Here's how the part is built. I have some questions about the finished solid (model axes, mm). Face numbers are marked on the shaded views. A direction names the side the tool comes from. Coordinates: 2 decimals unless noted, no trailing zeros. Write each loop counter-clockwise with the first axis right and the second up, starting at its lowest first coordinate (ties: lowest second). Pieces come first, ordered by that corner, then holes. Notation, with made-up numbers: M 79.5,-34.75 L 103.5,-34.75 A21 cw 103.5,-23.75 Z; hole C 76,1 d11. An arc over 180 degrees is marked long. Write each question's results on one line, items separated by ' | '. Start each with the question number.
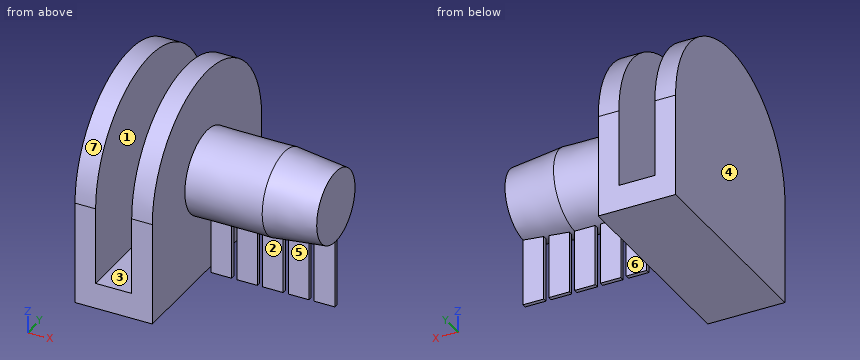
from build123d import *

# Parameters (mm, degrees)
BOX002004_W           = 4
BOX002004_H           = 0.8
BOX002004_DEPTH       = 13
BOX002003_W           = 4
BOX002003_H           = 0.8
BOX002003_DEPTH       = 13
BOX002002_W           = 4
BOX002002_H           = 0.8
BOX002002_DEPTH       = 13
BOX002001_W           = 4
BOX002001_H           = 0.8
BOX002001_DEPTH       = 13
BOX002_W              = 4
BOX002_H              = 0.8
BOX002_DEPTH          = 13
BOX001_W              = 36
BOX001_H              = 46
BOX001_DEPTH          = 7
CYLINDER001_R         = 20
CYLINDER001_DEPTH     = 15
BOX_W                 = 20
BOX_H                 = 40
BOX_DEPTH             = 15
FUSION002_PITCH_ANGLE = 90


with BuildPart() as support005:
    # Box002004 → Box002004 (new body)
    with BuildSketch(Plane(origin=(36, -0.4, -20), x_dir=(1, 0, 0), z_dir=(0, 0, 1))):
        with Locations((2, 0.4)):
            Rectangle(BOX002004_W, BOX002004_H)
    extrude(amount=BOX002004_DEPTH)


with BuildPart() as support004:
    # Box002003 → Box002003 (new body)
    with BuildSketch(Plane(origin=(31, -0.4, -20), x_dir=(1, 0, 0), z_dir=(0, 0, 1))):
        with Locations((2, 0.4)):
            Rectangle(BOX002003_W, BOX002003_H)
    extrude(amount=BOX002003_DEPTH)


with BuildPart() as support003:
    # Box002002 → Box002002 (new body)
    with BuildSketch(Plane(origin=(26, -0.4, -20), x_dir=(1, 0, 0), z_dir=(0, 0, 1))):
        with Locations((2, 0.4)):
            Rectangle(BOX002002_W, BOX002002_H)
    extrude(amount=BOX002002_DEPTH)


with BuildPart() as support002:
    # Box002001 → Box002001 (new body)
    with BuildSketch(Plane(origin=(21, -0.4, -20), x_dir=(1, 0, 0), z_dir=(0, 0, 1))):
        with Locations((2, 0.4)):
            Rectangle(BOX002001_W, BOX002001_H)
    extrude(amount=BOX002001_DEPTH)


with BuildPart() as support:
    # Box002 → Box002 (new body)
    with BuildSketch(Plane(origin=(16, -0.4, -20), x_dir=(1, 0, 0), z_dir=(0, 0, 1))):
        with Locations((2, 0.4)):
            Rectangle(BOX002_W, BOX002_H)
    extrude(amount=BOX002_DEPTH)

    # Fusion003: union Support002
    add(support002.part)

    # Fusion004: union Support003
    add(support003.part)

    # Fusion005: union Support004
    add(support004.part)

    # Fusion006: union Support005
    add(support005.part)


with BuildPart() as cone001:
    # Cone001 → Cone001 (revolve)
    with BuildSketch(Plane(origin=(0, 0, 30), x_dir=(1, 0, 0), z_dir=(0, -1, 0))):
        Polygon((0, 0), (8.09, 0), (7, 10), (0, 10), align=None)
    revolve(axis=Axis((0, 0, 30), (0, 0, 1)))


with BuildPart() as prise_male:
    # Cone → Cone (revolve)
    with BuildSketch(Plane(origin=(0, 0, 15), x_dir=(1, 0, 0), z_dir=(0, -1, 0))):
        Polygon((0, 0), (8.1, 0), (8.09, 15), (0, 15), align=None)
    revolve(axis=Axis((0, 0, 15), (0, 0, 1)))

    # Fusion001: union Cone001
    add(cone001.part)


with BuildPart() as trou:
    # Box001 → Box001 (new body)
    with BuildSketch(Plane(origin=(-21, -23, 4), x_dir=(1, 0, 0), z_dir=(0, 0, 1))):
        with Locations((18, 23)):
            Rectangle(BOX001_W, BOX001_H)
    extrude(amount=BOX001_DEPTH)


with BuildPart() as cylinder_corps:
    # Cylinder001 → Cylinder001 (new body)
    with BuildSketch(Plane.XY):
        Circle(CYLINDER001_R)
    extrude(amount=CYLINDER001_DEPTH)


with BuildPart() as obj1:
    # Box → Box (new body)
    with BuildSketch(Plane(origin=(0, -20, 0), x_dir=(1, 0, 0), z_dir=(0, 0, 1))):
        with Locations((10, 20)):
            Rectangle(BOX_W, BOX_H)
    extrude(amount=BOX_DEPTH)

    # Fusion: union Cylinder-corps
    add(cylinder_corps.part)

    # Cut: cut trou
    add(trou.part, mode=Mode.SUBTRACT)

    # Fusion002: union Prise male
    add(prise_male.part)


with BuildPart() as obj1_1:
    # Fusion002 pitch: moved
    add(obj1.part.rotate(Axis((0, 0, 0), (0, 1, 0)), FUSION002_PITCH_ANGLE))


with BuildPart() as obj1_2:
    # Fusion002 placement: moved
    add(obj1_1.part)

    # Fusion007: union Support
    add(support.part)


solid = obj1_2.part
1) I want a section at A-A, the plane z = 14. Write out the boundary of the cut face in (x, y), then the cut area to 3 significant figures.
2) Please list where these lines run through material, in increasing order: line 1 (X direction, y = 14, z = 6); line 2 (X direction, y = -1, z = 5); line 3 (Y direction, x = 24, z = 7). Write a range as [from, to].
3) I want a section at C-C, the plane y = -15. Write out the boundary of the cut face in (x, z), then the cut area to 3 significant figures.
4) For pin 1 Ø2 at (x, z) = (26.5, -11.5) entering from -Y; pin 2 Ø8 at (x, y) = (21.5, 1) entering from -Z; pin 3 Ø8 at (x, y) = (29.5, 8) entering from -Z; pin 4 Ø5 at (x, z) = (28.5, -9.5) entering from -Y, each with a flat end and sliding along its axis, tell me the tip position at first contact or that it passes through.
5) I want a section at D-D, the plane x = 13. Write out the boundary of the cut face in (y, z).
6) I want a section at B-B, the plane x = 8.5. Write out the boundary of the cut face in (y, z), then the cut area to 3 significant figures.
7) For the marked faces 5, 6 and 7, which set-ups out of +Z, -Z, +X, -X, +Y, -Y let a thin tool reach every point of the face, with its end or its side?
8) We'd pull the mould along X, two halves only. Please class the marked faces 1, 2, 3 and 4: pulls with the +X half, pulls with the -X half, needs draft (parallel to the pull), parting line crosses it, or undercut.
Output:
1) outline: M 0,-14.28 L 4,-14.28 L 4,14.28 L 0,14.28 Z; M 11,-14.28 L 15,-14.28 L 15,14.28 L 11,14.28 Z | area: 229 mm2
2) line 1: x = [0, 4], [11, 15] | line 2: x = [0, 4], [11, 40] | line 3: y = [-4.06, 4.06]
3) outline: M 0,-20 L 15,-20 L 15,13.23 L 11,13.23 L 11,-15 L 4,-15 L 4,13.23 L 0,13.23 Z | area: 301 mm2
4) pin 1: stops at y = -0.4 | pin 2: stops at z = -20 | pin 3: stops at z = -7.03 | pin 4: stops at y = -4.06
5) outline: M -20,-20 L 20,-20 L 20,0 A20 ccw -20,0 Z
6) outline: M -20,-20 L 20,-20 L 20,-15 L -20,-15 Z | area: 200 mm2
7) face 5: -Z, +X, -Y | face 6: -Z, +X, +Y | face 7: +Z, +X, -X
8) face 1: undercut | face 2: needs draft | face 3: undercut | face 4: pulls with the -X half
